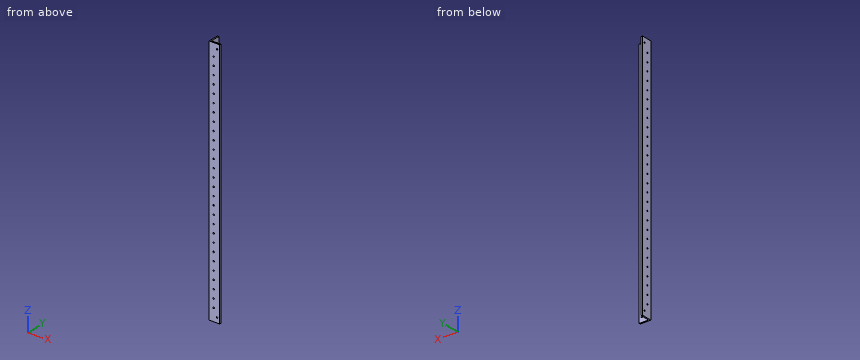
from build123d import *

# Parameters (mm, degrees)
BOSS_EXTRUDE1_DEPTH = 1219.2
FILLET1_R           = 0.4064
SKETCH4_W           = 1838.4
SKETCH4_H           = 103.278519729
CUT_EXTRUDE1_DEPTH  = 60
SKETCH5_W           = 2.838427027
SKETCH5_H           = 1.970979722
CUT_EXTRUDE2_DEPTH  = 700
SKETCH9_R           = 1.65
CUT_EXTRUDE5_DEPTH  = 20
SKETCH10_R          = 1.65
CUT_EXTRUDE6_DEPTH  = 20
SKETCH11_R          = 1.65
CUT_EXTRUDE7_DEPTH  = 70
SKETCH12_R          = 1.65
CUT_EXTRUDE8_DEPTH  = 70


with BuildPart() as part:
    # Sketch3 → Boss-Extrude1 (new, symmetric)
    with BuildSketch(Plane.XY):
        Polygon((3.175, 25.4), (0, 25.4), (0, 0), (25.4, 0), (25.4, 3.175), (3.175, 3.175), align=None)
    extrude(amount=BOSS_EXTRUDE1_DEPTH, both=True)

    # Fillet1
    fillet1_edges = [part.edges().sort_by_distance(p)[0] for p in [
        (3.175, 3.175, 0),
    ]]
    fillet(fillet1_edges, radius=FILLET1_R)

    # Sketch4 → Cut-Extrude1 (cut)
    with BuildSketch(Plane.ZY):
        with Locations((-300, -26.239259864)):
            Rectangle(SKETCH4_W, SKETCH4_H)
    extrude(amount=-CUT_EXTRUDE1_DEPTH, mode=Mode.SUBTRACT)

    # Sketch5 → Cut-Extrude2 (cut)
    with BuildSketch(Plane(origin=(0, 0, 619.2), x_dir=(-1, 0, 0), z_dir=(0, 0, -1))):
        with Locations((-4.594213514, 4.160489861)):
            Rectangle(SKETCH5_W, SKETCH5_H)
    extrude(amount=-CUT_EXTRUDE2_DEPTH, mode=Mode.SUBTRACT)

    # Sketch9 → Cut-Extrude5 (cut)
    with BuildSketch(Plane(origin=(3.175, 0, 0), x_dir=(0, 0, -1), z_dir=(1, 0, 0))):
        with Locations(Location((-649.2, 10.675, 0), (0, 0, 90))):
            Circle(SKETCH9_R)
        with Locations(Location((-669.2, 10.675, 0), (0, 0, 90))):
            Circle(SKETCH9_R)
        with Locations(Location((-689.2, 10.675, 0), (0, 0, 90))):
            Circle(SKETCH9_R)
        with Locations(Location((-709.2, 10.675, 0), (0, 0, 90))):
            Circle(SKETCH9_R)
        with Locations(Location((-729.2, 10.675, 0), (0, 0, 90))):
            Circle(SKETCH9_R)
        with Locations(Location((-749.2, 10.675, 0), (0, 0, 90))):
            Circle(SKETCH9_R)
        with Locations(Location((-769.2, 10.675, 0), (0, 0, 90))):
            Circle(SKETCH9_R)
        with Locations(Location((-789.2, 10.675, 0), (0, 0, 90))):
            Circle(SKETCH9_R)
        with Locations(Location((-809.2, 10.675, 0), (0, 0, 90))):
            Circle(SKETCH9_R)
        with Locations(Location((-829.2, 10.675, 0), (0, 0, 90))):
            Circle(SKETCH9_R)
        with Locations(Location((-849.2, 10.675, 0), (0, 0, 90))):
            Circle(SKETCH9_R)
        with Locations(Location((-869.2, 10.675, 0), (0, 0, 90))):
            Circle(SKETCH9_R)
        with Locations(Location((-889.2, 10.675, 0), (0, 0, 90))):
            Circle(SKETCH9_R)
        with Locations(Location((-909.2, 10.675, 0), (0, 0, 90))):
            Circle(SKETCH9_R)
        with Locations(Location((-929.2, 10.675, 0), (0, 0, 90))):
            Circle(SKETCH9_R)
        with Locations(Location((-949.2, 10.675, 0), (0, 0, 90))):
            Circle(SKETCH9_R)
        with Locations(Location((-969.2, 10.675, 0), (0, 0, 90))):
            Circle(SKETCH9_R)
        with Locations(Location((-989.2, 10.675, 0), (0, 0, 90))):
            Circle(SKETCH9_R)
        with Locations(Location((-1009.2, 10.675, 0), (0, 0, 90))):
            Circle(SKETCH9_R)
        with Locations(Location((-1029.2, 10.675, 0), (0, 0, 90))):
            Circle(SKETCH9_R)
        with Locations(Location((-1049.2, 10.675, 0), (0, 0, 90))):
            Circle(SKETCH9_R)
        with Locations(Location((-1069.2, 10.675, 0), (0, 0, 90))):
            Circle(SKETCH9_R)
        with Locations(Location((-1089.2, 10.675, 0), (0, 0, 90))):
            Circle(SKETCH9_R)
        with Locations(Location((-1109.2, 10.675, 0), (0, 0, 90))):
            Circle(SKETCH9_R)
        with Locations(Location((-1129.2, 10.675, 0), (0, 0, 90))):
            Circle(SKETCH9_R)
        with Locations(Location((-1149.2, 10.675, 0), (0, 0, 90))):
            Circle(SKETCH9_R)
        with Locations(Location((-1169.2, 10.675, 0), (0, 0, 90))):
            Circle(SKETCH9_R)
        with Locations(Location((-1189.2, 10.675, 0), (0, 0, 90))):
            Circle(SKETCH9_R)
    extrude(amount=-CUT_EXTRUDE5_DEPTH, mode=Mode.SUBTRACT)

    # Sketch10 → Cut-Extrude6 (cut)
    with BuildSketch(Plane(origin=(0, 3.175, 0), x_dir=(1, 0, 0), z_dir=(0, 1, 0))):
        with Locations(Location((10.675, -649.2, 0), (0, 0, 180))):
            Circle(SKETCH10_R)
        with Locations(Location((10.675, -669.2, 0), (0, 0, 180))):
            Circle(SKETCH10_R)
        with Locations(Location((10.675, -689.2, 0), (0, 0, 180))):
            Circle(SKETCH10_R)
        with Locations(Location((10.675, -709.2, 0), (0, 0, 180))):
            Circle(SKETCH10_R)
        with Locations(Location((10.675, -729.2, 0), (0, 0, 180))):
            Circle(SKETCH10_R)
        with Locations(Location((10.675, -749.2, 0), (0, 0, 180))):
            Circle(SKETCH10_R)
        with Locations(Location((10.675, -769.2, 0), (0, 0, 180))):
            Circle(SKETCH10_R)
        with Locations(Location((10.675, -789.2, 0), (0, 0, 180))):
            Circle(SKETCH10_R)
        with Locations(Location((10.675, -809.2, 0), (0, 0, 180))):
            Circle(SKETCH10_R)
        with Locations(Location((10.675, -829.2, 0), (0, 0, 180))):
            Circle(SKETCH10_R)
        with Locations(Location((10.675, -849.2, 0), (0, 0, 180))):
            Circle(SKETCH10_R)
        with Locations(Location((10.675, -869.2, 0), (0, 0, 180))):
            Circle(SKETCH10_R)
        with Locations(Location((10.675, -889.2, 0), (0, 0, 180))):
            Circle(SKETCH10_R)
        with Locations(Location((10.675, -909.2, 0), (0, 0, 180))):
            Circle(SKETCH10_R)
        with Locations(Location((10.675, -929.2, 0), (0, 0, 180))):
            Circle(SKETCH10_R)
        with Locations(Location((10.675, -949.2, 0), (0, 0, 180))):
            Circle(SKETCH10_R)
        with Locations(Location((10.675, -969.2, 0), (0, 0, 180))):
            Circle(SKETCH10_R)
        with Locations(Location((10.675, -989.2, 0), (0, 0, 180))):
            Circle(SKETCH10_R)
        with Locations(Location((10.675, -1009.2, 0), (0, 0, 180))):
            Circle(SKETCH10_R)
        with Locations(Location((10.675, -1029.2, 0), (0, 0, 180))):
            Circle(SKETCH10_R)
        with Locations(Location((10.675, -1049.2, 0), (0, 0, 180))):
            Circle(SKETCH10_R)
        with Locations(Location((10.675, -1069.2, 0), (0, 0, 180))):
            Circle(SKETCH10_R)
        with Locations(Location((10.675, -1089.2, 0), (0, 0, 180))):
            Circle(SKETCH10_R)
        with Locations(Location((10.675, -1109.2, 0), (0, 0, 180))):
            Circle(SKETCH10_R)
        with Locations(Location((10.675, -1129.2, 0), (0, 0, 180))):
            Circle(SKETCH10_R)
        with Locations(Location((10.675, -1149.2, 0), (0, 0, 180))):
            Circle(SKETCH10_R)
        with Locations(Location((10.675, -1169.2, 0), (0, 0, 180))):
            Circle(SKETCH10_R)
        with Locations(Location((10.675, -1189.2, 0), (0, 0, 180))):
            Circle(SKETCH10_R)
    extrude(amount=-CUT_EXTRUDE6_DEPTH, mode=Mode.SUBTRACT)

    # Sketch11 → Cut-Extrude7 (cut)
    with BuildSketch(Plane(origin=(0, 3.175, 0), x_dir=(1, 0, 0), z_dir=(0, 1, 0))):
        with Locations(Location((19.05, -1207.2366, 0), (0, 0, 180))):
            Circle(SKETCH11_R)
        with Locations(Location((19.05, -631.1634, 0), (0, 0, 180))):
            Circle(SKETCH11_R)
    extrude(amount=-CUT_EXTRUDE7_DEPTH, mode=Mode.SUBTRACT)

    # Sketch12 → Cut-Extrude8 (cut)
    with BuildSketch(Plane(origin=(3.175, 0, 0), x_dir=(0, 0, -1), z_dir=(1, 0, 0))):
        with Locations(Location((-1207.2366, 19.05, 0), (0, 0, 90))):
            Circle(SKETCH12_R)
        with Locations(Location((-631.1634, 19.05, 0), (0, 0, 90))):
            Circle(SKETCH12_R)
    extrude(amount=-CUT_EXTRUDE8_DEPTH, mode=Mode.SUBTRACT)


solid = part.part
Geometry check sheet. Reference: the model listing, model coordinates, mm. Coordinates: 2 decimals unless noted, no trailing zeros. Order: outer loops, then holes, each group sorted by start corner. A loop starts at its lowest first (then second) coordinate and runs counter-clockwise, first axis right, second up. Notation, with made-up numbers: (68, 6) - (90, 6) arc R24 ccw to (90, 35) - close; hole circle Ø9 at (83.5, 72). An arc over 180 degrees is marked (long way). Answer in a Markdown table with one row per item. Add a question column.
1) Gauge pin test, flat ends, axial feed: P1, Ø2.5, axis at y = 10.675, z = 849.2, coming from the +X side; P2, Ø12, axis at y = 17.5, z = 1051, coming from the +X side (3 decimals); P3, Ø5.5, axis at x = 10.675, z = 889.2, coming from the +Y side (3 decimals). Record the tip position at first contact, or that the pin passes through.
2) Material ranges on line 1 along Y through (x, z) = (0.9, 789.2) (3 decimals); line 2 along X through (y, z) = (21, 820.5) (3 decimals), recorded low to high. Write a range as [from, to].
3) Cross-section at A-A, the plane z = 1058. Record the cut outline in (x, y) (3 decimals).
Check result:
| question | item | result |
|---|---|---|
| 1 | P1 | passes through |
| 1 | P2 | stops at x = 3.175 |
| 1 | P3 | stops at y = 3.175 |
| 2 | line 1 | y = [0, 9.025], [12.325, 25.4] |
| 2 | line 2 | x = [0, 3.175] |
| 3 | outline | (0, 0) - (25.4, 0) - (25.4, 3.175) - (3.175, 3.175) - (3.175, 25.4) - (0, 25.4) - close |
